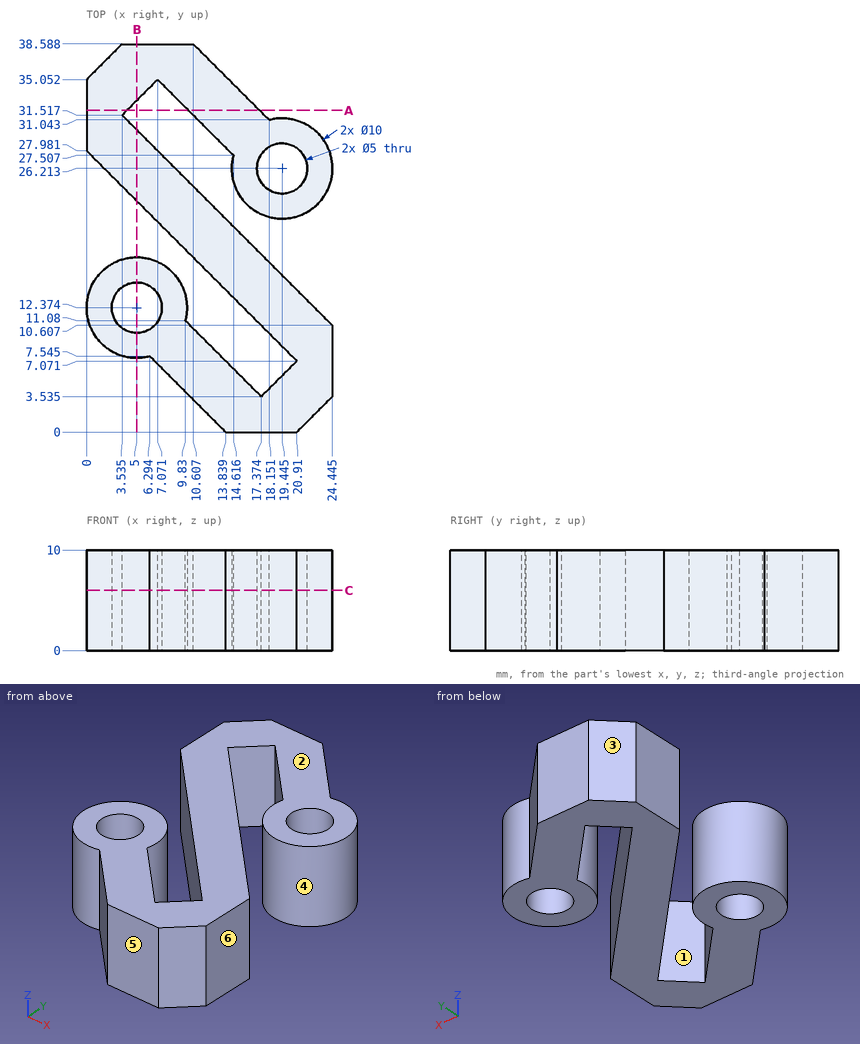
Can you work these out from the drawing? Everything is in mm from the part's minimum corner. A direction names the side the tool comes from. Give positions to 0.01 mm unless a question says otherwise; leave off trailing zeros. Order: outer loops, then holes, each group sorted by start corner. A loop starts at its lowest first (then second) coordinate and runs counter-clockwise, first axis right, second up. Notation, with made-up numbers: M -2,10 L 57,10 A27 ccw 57,26 Z; hole C -17.75,-16 d10. An arc over 180 degrees is marked long. One line per item, written item: value.
Item 1: If we section it at A-A on y = 32: Write out the boundary of the cut face in (x, z) (1 decimal).
Verdict:
outline: M 0,0 L 4,0 L 4,10 L 0,10 Z; M 10.1,0 L 17.2,0 L 17.2,10 L 10.1,10 Z
Item 2: If we mould it in two halves opening along Y, with no side actions, what happens to the marked faces 3, 4, 5 and 6? For each: pulls with the +Y half, pulls with the -Y half, needs draft (parallel to the pull), parting line crosses it, or undercut.
Verdict:
face 3: pulls with the +Y half
face 4: undercut
face 5: pulls with the -Y half
face 6: needs draft
Item 3: For the marked faces 1 and 2, which set-ups out of +Z, -Z, +X, -X, +Y, -Y let a thin tool reach every point of the face, with its end or its side?
Verdict:
face 1: +Z, -Z
face 2: +Z, +X, -X, +Y, -Y
Item 4: For pin 1 (1 mm diameter, centred on y = 22, z = 3.5, fed in from +X) (1 decimal); pin 2 (5 mm diameter, centred on y = 20.5, z = 6.5, fed in from +X) (1 decimal); pin 3 (4 mm diameter, centred on x = 15.5, z = 2, fed in from +Y) (1 decimal), each with a flat end and sliding along its axis, tell me the tip position at first contact or that it passes through.
Verdict:
pin 1: x = 22.8
pin 2: x = 23.3
pin 3: y = 35.7
Item 5: If we section it at B-B on x = 5: Write out the boundary of the cut face in (y, z) (1 decimal).
Verdict:
outline: M 7.4,0 L 9.9,0 L 9.9,10 L 7.4,10 Z; M 14.9,0 L 17.4,0 L 17.4,10 L 14.9,10 Z; M 23,0 L 30.1,0 L 30.1,10 L 23,10 Z; M 33,0 L 38.6,0 L 38.6,10 L 33,10 Z
Item 6: Please list where these lines run through material, in increasing order: line 1 (Y direction, x = 6.75, z = 8.25) (1 decimal); line 2 (X direction, y = 5, z = 1.75) (1 decimal); line 3 (X direction, y = 32, z = 4.25) (1 decimal).
Verdict:
line 1: 7.1 to 10.6, 14.2 to 17.1, 21.2 to 28.3, 34.7 to 38.6
line 2: 8.8 to 15.9, 18.8 to 24.4
line 3: 0 to 4, 10.1 to 17.2
Item 7: If we section it at C-C on z = 6: Write out the boundary of the cut face in (x, y) (1 decimal).
Verdict:
outline: M 0,28 L 20.9,7.1 L 17.4,3.5 L 9.8,11.1 A5 ccw long 6.3,7.5 L 13.8,0 L 20.9,0 L 24.4,3.5 L 24.4,10.6 L 3.5,31.5 L 7.1,35.1 L 14.6,27.5 A5 ccw long 18.2,31 L 10.6,38.6 L 3.5,38.6 L 0,35.1 Z; hole C 5,12.4 d5; hole C 19.4,26.2 d5
